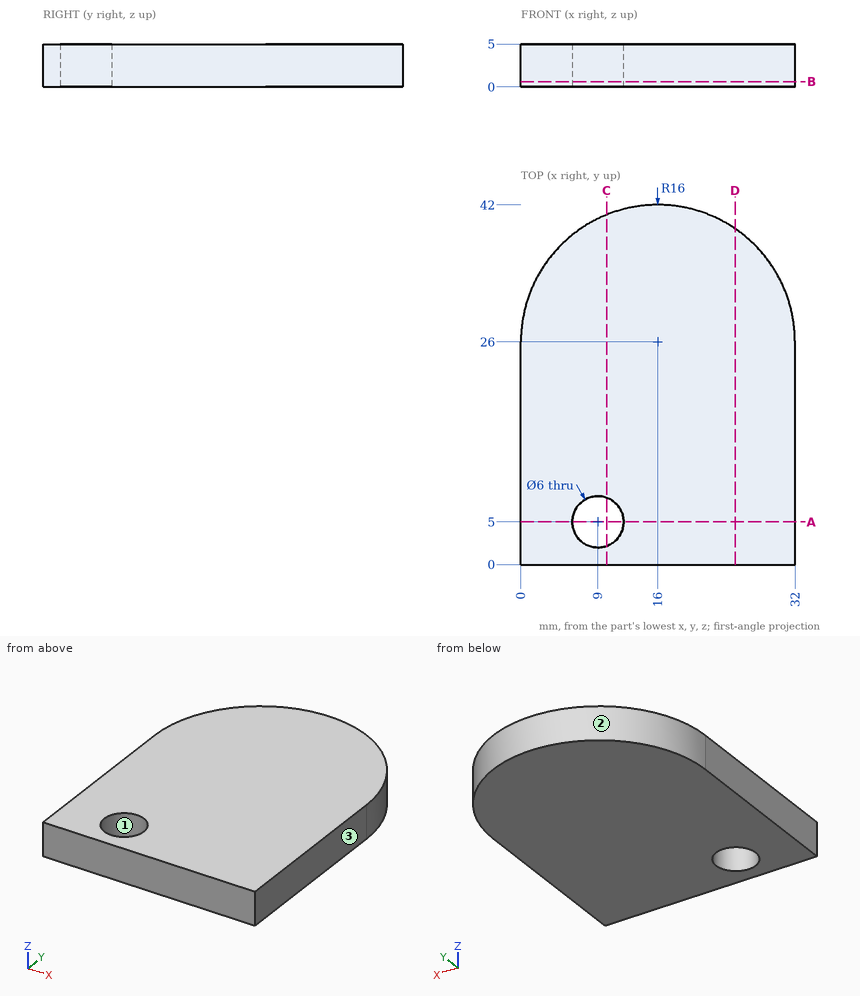
The figure shows three views and two pictorial views of one solid part (mm, origin at its lowest corner). Answer the questions. Round coordinates to 2 decimals unless told otherwise and drop trailing zeros. Loops run counter-clockwise (first coordinate to the right, second up) from the corner with the lowest first, then second, coordinate; pieces in that order, holes last. Notation, with made-up numbers: (38.25, -28.5) - (62.25, -28.5) arc R15 ccw to (62.25, -5.5) - close; hole circle Ø10 at (25, 21). An arc over 180 degrees is marked (long way). Use one line per item in the form item = value. Start each with the question number.
(1) Determine the mould class of the marked faces 1, 2 and 3 for opening direction X: +X half, -X half, draft (parallel to the pull), parting line (faces both ways), or undercut.
(2) A flat-ended cylindrical pin translates along its axis: P1, Ø1, axis at y = 35, z = 2.5, coming from the +X side. Find the tip coordinate at first contact, or state that the pin passes through.
(3) Find section B-B on z = 0.6. Determine the outline of the cut face in (x, y).
(4) Find section A-A on y = 5. Determine the outline of the cut face in (x, z), and give its area (3 significant figures).
(5) Find section C-C on x = 10. Determine the outline of the cut face in (y, z).
(6) Consider line 1 (X direction, y = 5, z = 3.8); line 2 (Y direction, x = 9, z = 1.65); line 3 (X direction, y = 6.5, z = 1.6). Determine where each line is inside the solid, lowest interval first.
(7) Find section D-D on x = 25. Determine the outline of the cut face in (y, z), and give its area (3 significant figures).
Answer list:
q1.face_1 = undercut
q1.face_2 = parting line
q1.face_3 = +X half
q2.P1 = 29.56
q3.outline = (0, 0) - (32, 0) - (32, 26) arc R16 ccw to (0, 26) - close; hole circle Ø6 at (9, 5)
q4.outline = (0, 0) - (6, 0) - (6, 5) - (0, 5) - close; (12, 0) - (32, 0) - (32, 5) - (12, 5) - close
q4.area = 130 mm^2
q5.outline = (0, 0) - (2.17, 0) - (2.17, 5) - (0, 5) - close; (7.83, 0) - (40.83, 0) - (40.83, 5) - (7.83, 5) - close
q6.line_1 = 0 to 6, 12 to 32
q6.line_2 = 0 to 2, 8 to 40.39
q6.line_3 = 0 to 6.4, 11.6 to 32
q7.outline = (0, 0) - (39.23, 0) - (39.23, 5) - (0, 5) - close
q7.area = 196 mm^2
